Read the model definition and answer for the solid it produces. Units are mm, in the model's axes. A direction names the side the tool comes from. Coordinates: 2 decimals unless noted, no trailing zeros. Write each loop counter-clockwise with the first axis right and the second up, starting at its lowest first coordinate (ties: lowest second). Pieces come first, ordered by that corner, then holes. Notation, with made-up numbers: (40.25, 50.5) -> (49.25, 50.5) arc R27 cw to (49.25, 72.5) -> close; hole circle Ø9 at (-30, -28). An arc over 180 degrees is marked (long way). Answer in a Markdown table with one row per item. Add a question column.
Item 1: Given pin 1 Ø3 at (x, z) = (-4.5, 48.5) entering from -Y; pin 2 Ø1 at (x, y) = (-27, -128) entering from -Z; pin 3 Ø9 at (y, z) = (18.5, -106) entering from -X, each flat-ended and moving along its own axis, determine where each tip first touches the part or whether it passes through.
Item 2: Section C-C on z = 254 is taken. Write down the section's boundary in (x, y).
Item 3: Section A-A on y = -27.5 is taken. Write down the section's boundary in (x, z), then the cut area to 3 significant figures.
Item 4: For a pull along Y with two mould halves and no side action, classify faces 1 (the face through (-15, 38, -4)), 2 (the face through (-9, 19, -4)), 3 (the face through (-15.338, 20.915, -258.619)), 4 (the face through (-15, -84, 215.9)) as +Y half, -Y half, draft (parallel to the pull), parting line (faces both ways), or undercut.
Item 5: Section D-D on z = -244 is taken. Write down the section's boundary in (x, y).
Item 6: Which of the six approach directions +Z, -Z, +X, -X, +Y, -Y give full straight-line access (tool end or side, diameter ignored) to faces 5 (the face through (-21.5, 19, -4)), 6 (the face through (-15, 0, 247)), 7 (the face through (-15, -84, -215.9)), 8 (the face through (-19, -170, 208)), 9 (the face through (-15, -84, -195.9))?
Item 7: Straight lines are drawn through the part: line 1 (Z direction, x = -15, y = -97.5); line 2 (Z direction, x = -15.5, y = 19); line 3 (Y direction, x = -16.5, z = 254). For each, find the intervals that lie inside material, in ascending order. Write a range as from..to.
Item 8: Section B-B on y = 19 is taken. Write down the section's boundary in (x, z), then the cut area to 3 significant figures.
Autodesk Inventor part; units mm, degrees
ref_plane "YZ Plane" through (0, 0, 0) normal (1, 0, 0) x (0, 1, 0)
ref_plane "XZ Plane" through (0, 0, 0) normal (0, 1, 0) x (-1, 0, 0)
ref_plane "XY Plane" through (0, 0, 0) normal (0, 0, 1) x (1, 0, 0)
sketch "Sketch1" plane through (0, 0, 0) normal (0, 0, 1) x (1, 0, 0)
  line L0 (0, 0) -> (-30.5, 0)
  line L1 (-30.5, 0) -> (-30.5, 38)
  line L2 (-30.5, 38) -> (0, 38)
  line L3 (0, 38) -> (0, 0)
  line L4 (0, 0) -> (0, 7)
  line L5 (0, 38) -> (0, 31)
  line L6 (0, 31) -> (-6, 31)
  line L7 (0, 7) -> (-6, 7)
  line L8 (-9, 10) -> (-9, 28)
  line L9 (-30.5, 38) -> (-30.5, 31)
  line L10 (-30.5, 31) -> (-24.5, 31)
  line L11 (-21.5, 28) -> (-21.5, 10)
  line L12 (-30.5, 0) -> (-30.5, 7)
  line L13 (-30.5, 7) -> (-24.5, 7)
  arc A0 (-6, 31) -> (-9, 28) centre (-6, 28) ccw
  arc A1 (-9, 10) -> (-6, 7) centre (-6, 10) ccw
  arc A2 (-21.5, 28) -> (-24.5, 31) centre (-24.5, 28) ccw
  arc A3 (-24.5, 7) -> (-21.5, 10) centre (-24.5, 10) ccw
  point P0 (-9, 31)
  point P1 (-21.5, 31)
  dimension "d0" = 30.5
  dimension "d1" = 38
  dimension "d2" = 7
  dimension "d3" = 7
  dimension "d4" = 9
  dimension "d6" = 7
  dimension "d7" = 9
  dimension "d8" = 7
  dimension "d9" = 3
  dimension "d11" = 3
extrude "Extrusion1" add sketch "Sketch1" along normal mid plane 558.8 contours L0 L1 L13 A3 L11 A2 L10 L2 L3 L6 A0 L8 A1 L7
hole "Hole1" at (-9, 19, 254) direction (-1, 0, 0) diameter 10 depth 25
hole "Hole2" at (-9, 19, -254) direction (-1, 0, 0) diameter 10 depth 25 tip angle 118
sketch "Sketch2" plane through (-30.5, 0, 279.4) normal (0, -1, 0) x (1, 0, 0)
  line L0 (0, 0) -> (30.5, 0)
  line L1 (15.25, 0) -> (15.25, -63.5)
  line L2 (15.25, -63.5) -> (0, -63.5)
  line L3 (0, -558.8) -> (0, 0)
  line L4 (15.25, -63.5) -> (30.5, -63.5)
  line L5 (30.5, -63.5) -> (30.5, -83.5)
  line L6 (30.5, -558.8) -> (30.5, 0)
  line L7 (30.5, -83.5) -> (0, -83.5)
  line L8 (0, -83.5) -> (0, -63.5)
  line L9 (30.5, -558.8) -> (0, -558.8)
  line L10 (15.25, -558.8) -> (15.25, -495.3)
  line L11 (15.25, -495.3) -> (30.5, -495.3)
  line L12 (15.25, -495.3) -> (0, -495.3)
  line L13 (0, -495.3) -> (0, -475.3)
  line L14 (0, -475.3) -> (30.5, -475.3)
  line L15 (30.5, -475.3) -> (30.5, -495.3)
  point P0 (30.5, -279.4)
  dimension "d33" = 63.5
  dimension "d34" = 20
  dimension "d35" = 30.5
  dimension "d36" = 63.5
  dimension "d37" = 20
extrude "Extrusion2" add sketch "Sketch2" along normal blind 170 contours L2 L4 L5 L7 L3 | L14 L6 L11 L12 L3
sketch "Sketch5" plane through (-30.5, 38, 279.4) normal (0, 1, 0) x (1, 0, 0)
  point P0 (30.5, 279.4)
sketch "Sketch8" plane through (-30.5, -170, 279.4) normal (0, -1, 0) x (1, 0, 0)
  line L0 (30.5, -83.5) -> (30.5, -63.5)
  line L1 (30.5, -63.5) -> (0, -63.5)
  point P0 (30.5, -279.4)
  point P1 (15.5, -73.5)
  dimension "d72" = 15
  dimension "d73" = 10
hole "Hole5" at (-15, -170, 205.9) direction (0, 1, 0) diameter 8.647 end through all
sketch "Sketch9" plane through (-30.5, -170, 279.4) normal (0, -1, 0) x (1, 0, 0)
  line L0 (30.5, -495.3) -> (30.5, -475.3)
  line L1 (30.5, -475.3) -> (0, -475.3)
  point P0 (30.5, -279.4)
  point P1 (15.5, -485.3)
  dimension "d81" = 15
  dimension "d82" = 10
hole "Hole6" at (-15, -170, -205.9) direction (0, 1, 0) diameter 8.647 end through all
properties part number "BarraEx"
Results below:
| question | item | result |
|---|---|---|
| 1 | pin 1 | stops at y = 0 |
| 1 | pin 2 | stops at z = -215.9 |
| 1 | pin 3 | stops at x = -21.5 |
| 2 | outline | (-30.5, 0) -> (0, 0) -> (0, 7) -> (-6, 7) arc R3 cw to (-9, 10) -> (-9, 14) -> (-21.5, 14) -> (-21.5, 10) arc R3 cw to (-24.5, 7) -> (-30.5, 7) -> close; (-30.5, 31) -> (-24.5, 31) arc R3 cw to (-21.5, 28) -> (-21.5, 24) -> (-9, 24) -> (-9, 28) arc R3 cw to (-6, 31) -> (0, 31) -> (0, 38) -> (-30.5, 38) -> close |
| 3 | outline | (-30.5, -215.9) -> (0, -215.9) -> (0, -195.9) -> (-30.5, -195.9) -> close; (-30.5, 195.9) -> (0, 195.9) -> (0, 215.9) -> (-30.5, 215.9) -> close; hole circle Ø8.65 at (-15, -205.9); hole circle Ø8.65 at (-15, 205.9) |
| 3 | area | 1,100 mm2 |
| 4 | face 1 | +Y half |
| 4 | face 2 | undercut |
| 4 | face 3 | undercut |
| 4 | face 4 | draft |
| 5 | outline | (-30.5, 0) -> (0, 0) -> (0, 7) -> (-6, 7) arc R3 cw to (-9, 10) -> (-9, 28) arc R3 cw to (-6, 31) -> (0, 31) -> (0, 38) -> (-30.5, 38) -> (-30.5, 31) -> (-24.5, 31) arc R3 cw to (-21.5, 28) -> (-21.5, 10) arc R3 cw to (-24.5, 7) -> (-30.5, 7) -> close |
| 6 | face 5 | +Z, -Z, -X |
| 6 | face 6 | +Z, +X, -X, -Y |
| 6 | face 7 | -Z, +X, -X, -Y |
| 6 | face 8 | +Z, -Z, +X, -X, -Y |
| 6 | face 9 | +X, -X, -Y |
| 7 | line 1 | z = -215.9..-210.22, -201.58..-195.9, 195.9..201.58, 210.22..215.9 |
| 7 | line 2 | z = -279.4..-259, -249..-210.19, -201.61..201.61, 210.19..249, 259..279.4 |
| 7 | line 3 | y = 0..14, 24..38 |
| 8 | outline | (-21.5, -279.4) -> (-9, -279.4) -> (-9, -259) -> (-21.5, -259) -> close; (-21.5, -249) -> (-9, -249) -> (-9, 249) -> (-21.5, 249) -> close; (-21.5, 259) -> (-9, 259) -> (-9, 279.4) -> (-21.5, 279.4) -> close; hole circle Ø8.65 at (-15, -205.9); hole circle Ø8.65 at (-15, 205.9) |
| 8 | area | 6,620 mm2 |
